Model file for the job. Use its own axes, mm. Give positions to 0.01 mm unless a question says otherwise; leave off trailing zeros. Write each loop counter-clockwise with the first axis right and the second up, starting at its lowest first coordinate (ties: lowest second). Pieces come first, ordered by that corner, then holes. Notation, with made-up numbers: (60.5, 25.5) - (84.5, 25.5) arc R21 ccw to (84.5, 45.5) - close; hole circle Ø8 at (-14.75, 49). An arc over 180 degrees is marked (long way). Use CSV: the item, a comma, the result in double quotes.
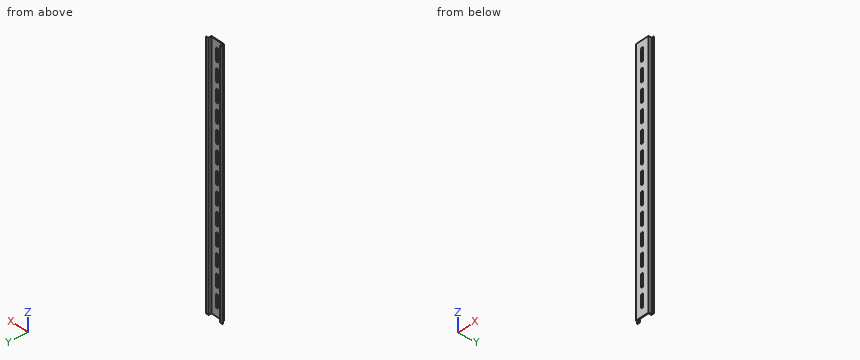
from build123d import *

# Parameters (mm, degrees)
BOSS_EXTRUDE1_DEPTH    = 242.5
FILLET1_R              = 0.5
SKETCH2_W              = 4.5
SKETCH2_H              = 25
CUT_EXTRUDE1_DEPTH     = 244.199794408
FILLET2_R              = 2
LPATTERN1_COUNT        = 13
LPATTERN1_PITCH        = 36
FILLET2_OF_LPATTERN1_R = 2


with BuildPart() as part:
    # Sketch1 → Boss-Extrude1 (new, symmetric)
    with BuildSketch(Plane.XY):
        Polygon((-13.5, 0), (13.5, 0), (13.5, 6.3), (17.5, 6.3), (17.5, 7.3), (12, 7.3), (12, 1.5), (-12, 1.5), (-12, 7.3), (-17.5, 7.3), (-17.5, 6.3), (-13.5, 6.3), align=None)
    extrude(amount=BOSS_EXTRUDE1_DEPTH, both=True)

    # Fillet1
    fillet1_edges = [part.edges().sort_by_distance(p)[0] for p in [
        (-13.5, 6.3, 0),
        (-12, 7.3, 0),
        (-12, 1.5, 0),
        (12, 1.5, 0),
        (12, 7.3, 0),
        (13.5, 6.3, 0),
        (13.5, 0, 0),
        (-13.5, 0, 0),
    ]]
    fillet(fillet1_edges, radius=FILLET1_R)

    # Sketch2 → Cut-Extrude1 (cut, through all)
    with BuildSketch(Plane(origin=(0, 1.5, 0), x_dir=(1, 0, 0), z_dir=(0, 1, 0))):
        with Locations((0, 215)):
            Rectangle(SKETCH2_W, SKETCH2_H)
    cut_extrude1 = extrude(amount=-CUT_EXTRUDE1_DEPTH, mode=Mode.SUBTRACT)

    # Fillet2
    fillet2_edges = [part.edges().sort_by_distance(p)[0] for p in [
        (2.25, 0.75, -227.5),
        (2.25, 0.75, -202.5),
        (-2.25, 0.75, -202.5),
        (-2.25, 0.75, -227.5),
    ]]
    fillet(fillet2_edges, radius=FILLET2_R)

    # LPattern1: Cut-Extrude1 ×13
    with Locations(*[(0, 0, i * LPATTERN1_PITCH) for i in range(1, LPATTERN1_COUNT)]):
        add(cut_extrude1, mode=Mode.SUBTRACT)

    # Fillet2 of LPattern1
    fillet2_of_lpattern1_edges = [part.edges().sort_by_distance(p)[0] for p in [
        (2.25, 0.75, -191.5),
        (2.25, 0.75, -166.5),
        (-2.25, 0.75, -166.5),
        (-2.25, 0.75, -191.5),
        (2.25, 0.75, -155.5),
        (2.25, 0.75, -130.5),
        (-2.25, 0.75, -130.5),
        (-2.25, 0.75, -155.5),
        (2.25, 0.75, -119.5),
        (2.25, 0.75, -94.5),
        (-2.25, 0.75, -94.5),
        (-2.25, 0.75, -119.5),
        (2.25, 0.75, -83.5),
        (2.25, 0.75, -58.5),
        (-2.25, 0.75, -58.5),
        (-2.25, 0.75, -83.5),
        (2.25, 0.75, -47.5),
        (2.25, 0.75, -22.5),
        (-2.25, 0.75, -22.5),
        (-2.25, 0.75, -47.5),
        (2.25, 0.75, -11.5),
        (2.25, 0.75, 13.5),
        (-2.25, 0.75, 13.5),
        (-2.25, 0.75, -11.5),
        (2.25, 0.75, 24.5),
        (2.25, 0.75, 49.5),
        (-2.25, 0.75, 49.5),
        (-2.25, 0.75, 24.5),
        (2.25, 0.75, 60.5),
        (2.25, 0.75, 85.5),
        (-2.25, 0.75, 85.5),
        (-2.25, 0.75, 60.5),
        (2.25, 0.75, 96.5),
        (2.25, 0.75, 121.5),
        (-2.25, 0.75, 121.5),
        (-2.25, 0.75, 96.5),
        (2.25, 0.75, 132.5),
        (2.25, 0.75, 157.5),
        (-2.25, 0.75, 157.5),
        (-2.25, 0.75, 132.5),
        (2.25, 0.75, 168.5),
        (2.25, 0.75, 193.5),
        (-2.25, 0.75, 193.5),
        (-2.25, 0.75, 168.5),
        (2.25, 0.75, 204.5),
        (2.25, 0.75, 229.5),
        (-2.25, 0.75, 229.5),
        (-2.25, 0.75, 204.5),
    ]]
    fillet(fillet2_of_lpattern1_edges, radius=FILLET2_OF_LPATTERN1_R)


solid = part.part
(1) Saw through at B-B, the plane x = 7.5. List the corners of the cut face in (y, z).
Checked values:
outline,"(0, -242.5) - (1.5, -242.5) - (1.5, 242.5) - (0, 242.5) - close"
(2) Flat gauge pins, fed straight in: P1, Ø0.8, axis at y = 0.5, z = -217, coming from the +X side; P2, Ø4, axis at x = -1.5, z = -140, coming from the +Y side; P3, Ø0.8, axis at y = 0.5, z = -144, coming from the -X side. Where does each tip first touch, or does it go through?
Checked values:
P1,"stops at x = 13.5"
P2,"stops at y = 1.5"
P3,"stops at x = -13.5"
(3) Saw through at A-A, the plane z = 71. List the corners of the cut face in (x, y), then the cut area to 4 significant figures.
Checked values:
outline,"(-17.5, 6.3) - (-14, 6.3) arc R0.5 cw to (-13.5, 5.8) - (-13.5, 0.5) arc R0.5 ccw to (-13, 0) - (-2.25, 0) - (-2.25, 1.5) - (-11.5, 1.5) arc R0.5 cw to (-12, 2) - (-12, 6.8) arc R0.5 ccw to (-12.5, 7.3) - (-17.5, 7.3) - close; (2.25, 0) - (13, 0) arc R0.5 ccw to (13.5, 0.5) - (13.5, 5.8) arc R0.5 cw to (14, 6.3) - (17.5, 6.3) - (17.5, 7.3) - (12.5, 7.3) arc R0.5 ccw to (12, 6.8) - (12, 2) arc R0.5 cw to (11.5, 1.5) - (2.25, 1.5) - close"
area,"59.15 mm^2"
(4) Wall check: probe 1 along X at (y, z) = (5, 129.5); probe 2 along X at (y, z) = (1.75, 200); probe 3 along Y at (x, z) = (-0.5, -92.5). Give the ranges that are in metal, low to high. Write a range as [from, to].
Checked values:
probe 1,"x = [-13.5, -12], [12, 13.5]"
probe 2,"x = [-13.5, -11.93], [11.93, 13.5]"
probe 3,"y = [0, 1.5]"
